Model file for the job. Use its own axes, mm. A direction names the side the tool comes from. Coordinates: 2 decimals unless noted, no trailing zeros. Write each loop counter-clockwise with the first axis right and the second up, starting at its lowest first coordinate (ties: lowest second). Pieces come first, ordered by that corner, then holes. Notation, with made-up numbers: (67, -8) - (119, -8) arc R33 ccw to (119, 28) - close; hole circle Ø7 at (-12.75, 58). An arc over 180 degrees is marked (long way). Put each result on its own line as item: value. Start each with the question number.
1. Saw through at A-A, the plane x = -61. Write the cut outline in (y, z), plus the area to 3 significant figures.
2. Which spindle directions (+Z, -Z, +X, -X, +Y, -Y) get a long thin tool onto all of the face, cutting with end or side? Do faces 1 (the face through (86.358, 3.433, -10.902)), 2 (the face through (-1, 21.59, 24)), 3 (the face through (-90.7, -9.9, -1.5)), 4 (the face through (-1, 24, -21.59)), 5 (the face through (85.09, 12, 0)). Say none if no direction does.
3. Saw through at B-B, the plane y = 0. Write the cut outline in (x, z) (3 decimals), plus the area to 3 significant figures.
4. Saw through at C-C, the plane y = -7. Write the cut outline in (x, z).
5. Pull direction Y, two halves, no side cores. Call faces 6 (the face through (0, -25.4, 23)), 7 (the face through (-93.941, 0, -13)), 8 (the face through (0, 25.4, 23)), 9 (the face through (-90.7, 9.9, 1.5)): released by +Y, released by -Y, zero draft, split by the parting line, or undercut.
6. Drop flat-ended pins along their axis: P1, Ø8, axis at x = -46, z = -16.5, coming from the +Y side; P2, Ø4, axis at y = 19.5, z = -11.5, coming from the -X side. Give the stop position or say it passes through.
7. Drill centre lines: L1, parallel to Y at x = 86.35, z = 0 (3 decimals); L2, parallel to X at y = 13.5, z = -4; L3, parallel to X at y = -13, z = 2. Where is each one in solid material? Low to high. Write a range as from..to.
```python
from build123d import *

# Parameters (mm, degrees)
SKETCH2_W           = 175.181977678
SKETCH2_H           = 50.8
BOSS_EXTRUDE1_DEPTH = 25.4
SKETCH8_R           = 11.43
SKETCH8_R_2         = 1.27
CUT_EXTRUDE3_DEPTH  = 12.7
SKETCH10_W          = 170.18
SKETCH10_H          = 43.18
CUT_EXTRUDE5_DEPTH  = 51.8
SKETCH11_R          = 3.175
BOSS_EXTRUDE2_DEPTH = 6.35
CIRPATTERN2_COUNT   = 4
CIRPATTERN3_COUNT   = 2
CIRPATTERN3_ANGLE   = 90


with BuildPart() as part:
    # Sketch2 → Boss-Extrude1 (new body, symmetric)
    with BuildSketch(Plane.XY):
        Rectangle(SKETCH2_W, SKETCH2_H)
    extrude(amount=BOSS_EXTRUDE1_DEPTH, both=True)

    # Sketch8 → Cut-Extrude3 (cut)
    with BuildSketch(Plane(origin=(87.590988839, 0, 0), x_dir=(0, 0, -1), z_dir=(1, 0, 0))):
        Circle(SKETCH8_R)
        with Locations((0, 15.875)):
            Circle(SKETCH8_R_2)
        with Locations((0, -15.875)):
            Circle(SKETCH8_R_2)
    extrude(amount=-CUT_EXTRUDE3_DEPTH, mode=Mode.SUBTRACT)

    # Sketch10 → Cut-Extrude5 (cut, through all)
    with BuildSketch(Plane(origin=(0, 25.4, 0), x_dir=(1, 0, 0), z_dir=(0, 1, 0))):
        Rectangle(SKETCH10_W, SKETCH10_H)
    cut_extrude5 = extrude(amount=-CUT_EXTRUDE5_DEPTH, mode=Mode.SUBTRACT)

    # Sketch11 → Boss-Extrude2 (add)
    with BuildSketch(Plane.ZY.offset(87.590988839)):
        with Locations((0, 12.7)):
            Circle(SKETCH11_R)
    boss_extrude2 = extrude(amount=BOSS_EXTRUDE2_DEPTH)

    # CirPattern2: Boss-Extrude2 ×4 about axis
    cirpattern2_axis = Axis((0, 0, 0), (1, 0, 0))
    for i in range(1, CIRPATTERN2_COUNT):
        add(boss_extrude2.rotate(cirpattern2_axis, i * 360 / CIRPATTERN2_COUNT))

    # CirPattern3: Cut-Extrude5 ×2 about axis
    cirpattern3_axis = Axis((74.890988839, 0, 0), (1, 0, 0))
    for i in range(1, CIRPATTERN3_COUNT):
        add(cut_extrude5.rotate(cirpattern3_axis, i * CIRPATTERN3_ANGLE / (CIRPATTERN3_COUNT - 1)), mode=Mode.SUBTRACT)


solid = part.part
```
Final values:
1. outline: (-25.4, -25.4) - (-21.59, -25.4) - (-21.59, -21.59) - (-25.4, -21.59) - close; (-25.4, 21.59) - (-21.59, 21.59) - (-21.59, 25.4) - (-25.4, 25.4) - close; (21.59, -25.4) - (25.4, -25.4) - (25.4, -21.59) - (21.59, -21.59) - close; (21.59, 21.59) - (25.4, 21.59) - (25.4, 25.4) - (21.59, 25.4) - close
1. area: 58.1 mm²
2. face 1: +X
2. face 2: +Z, -Z
2. face 3: -X
2. face 4: +Y, -Y
2. face 5: none
3. outline: (-93.941, -15.875) - (-87.591, -15.875) - (-87.591, -25.4) - (-85.09, -25.4) - (-85.09, 25.4) - (-87.591, 25.4) - (-87.591, 15.875) - (-93.941, 15.875) - (-93.941, 9.525) - (-87.591, 9.525) - (-87.591, -9.525) - (-93.941, -9.525) - close; (85.09, -25.4) - (87.591, -25.4) - (87.591, -11.43) - (85.09, -11.43) - close; (85.09, 11.43) - (87.591, 11.43) - (87.591, 25.4) - (85.09, 25.4) - close
3. area: 278 mm²
4. outline: (-87.59, -25.4) - (-85.09, -25.4) - (-85.09, 25.4) - (-87.59, 25.4) - close; (85.09, -25.4) - (87.59, -25.4) - (87.59, -9.04) - (85.09, -9.04) - close; (85.09, 9.04) - (87.59, 9.04) - (87.59, 25.4) - (85.09, 25.4) - close
5. face 6: released by -Y
5. face 7: zero draft
5. face 8: released by +Y
5. face 9: undercut
6. P1: passes through
6. P2: stops at x = -87.59
7. L1: y = -25.4..-17.145, -14.605..-11.43, 11.43..14.605, 17.145..25.4
7. L2: x = -87.59..-85.09, 85.09..87.59
7. L3: x = -93.94..-85.09, 85.09..87.59
